Verification items for the finished model (mm, model axes). A direction names the side the tool comes from. Give positions to 0.01 mm unless a question says otherwise; leave off trailing zeros.
from build123d import *

# Parameters (mm, degrees)
SKETCH_2_R      = 2.5
EXTRUDE_1_DEPTH = 300


with BuildPart() as part:
    # 草图2 → 凸台-拉伸1 (new body)
    with BuildSketch(Plane.XY):
        with BuildLine():
            Line((-5.825824942, 5.993206118), (-5.825824942, 0.914526462))
            Line((-5.825824942, 0.914526462), (-8.786485114, -2.04613371))
            Line((-8.786485114, -2.04613371), (-10.425824942, -2.04613371))
            Line((-10.425824942, -2.04613371), (-10.425824942, 0.35386629))
            Line((-10.425824942, 0.35386629), (-11.425824942, 0.35386629))
            Line((-11.425824942, 0.35386629), (-11.425824942, -0.14613371))
            Line((-11.425824942, -0.14613371), (-12.225824942, -0.14613371))
            Line((-12.225824942, -0.14613371), (-12.225824942, -5.04613371))
            ThreePointArc((-12.225824942, -5.04613371), (-11.786485114, -6.106793882), (-10.725824942, -6.54613371))
            Line((-10.725824942, -6.54613371), (-5.825824942, -6.54613371))
            Line((-5.825824942, -6.54613371), (-5.825824942, -5.74613371))
            Line((-5.825824942, -5.74613371), (-5.325824942, -5.74613371))
            Line((-5.325824942, -5.74613371), (-5.325824942, -4.74613371))
            Line((-5.325824942, -4.74613371), (-7.725824942, -4.74613371))
            Line((-7.725824942, -4.74613371), (-7.725824942, -3.106793882))
            Line((-7.725824942, -3.106793882), (-4.765164771, -0.14613371))
            Line((-4.765164771, -0.14613371), (0.313514886, -0.14613371))
            Line((0.313514886, -0.14613371), (3.274175058, -3.106793882))
            Line((3.274175058, -3.106793882), (3.274175058, -4.74613371))
            Line((3.274175058, -4.74613371), (0.874175058, -4.74613371))
            Line((0.874175058, -4.74613371), (0.874175058, -5.74613371))
            Line((0.874175058, -5.74613371), (1.374175058, -5.74613371))
            Line((1.374175058, -5.74613371), (1.374175058, -6.54613371))
            Line((1.374175058, -6.54613371), (6.274175058, -6.54613371))
            ThreePointArc((6.274175058, -6.54613371), (7.334835229, -6.106793882), (7.774175058, -5.04613371))
            Line((7.774175058, -5.04613371), (7.774175058, -0.14613371))
            Line((7.774175058, -0.14613371), (6.974175058, -0.14613371))
            Line((6.974175058, -0.14613371), (6.974175058, 0.35386629))
            Line((6.974175058, 0.35386629), (5.974175058, 0.35386629))
            Line((5.974175058, 0.35386629), (5.974175058, -2.04613371))
            Line((5.974175058, -2.04613371), (4.334835229, -2.04613371))
            Line((4.334835229, -2.04613371), (1.374175058, 0.914526462))
            Line((1.374175058, 0.914526462), (1.374175058, 5.993206118))
            Line((1.374175058, 5.993206118), (4.334835229, 8.95386629))
            Line((4.334835229, 8.95386629), (5.974175058, 8.95386629))
            Line((5.974175058, 8.95386629), (5.974175058, 6.55386629))
            Line((5.974175058, 6.55386629), (6.974175058, 6.55386629))
            Line((6.974175058, 6.55386629), (6.974175058, 7.05386629))
            Line((6.974175058, 7.05386629), (7.774175058, 7.05386629))
            Line((7.774175058, 7.05386629), (7.774175058, 11.95386629))
            ThreePointArc((7.774175058, 11.95386629), (7.334835229, 13.014526462), (6.274175058, 13.45386629))
            Line((6.274175058, 13.45386629), (1.374175058, 13.45386629))
            Line((1.374175058, 13.45386629), (1.374175058, 12.65386629))
            Line((1.374175058, 12.65386629), (0.874175058, 12.65386629))
            Line((0.874175058, 12.65386629), (0.874175058, 11.65386629))
            Line((0.874175058, 11.65386629), (3.274175058, 11.65386629))
            Line((3.274175058, 11.65386629), (3.274175058, 10.014526462))
            Line((3.274175058, 10.014526462), (0.313514886, 7.05386629))
            Line((0.313514886, 7.05386629), (-4.765164771, 7.05386629))
            Line((-4.765164771, 7.05386629), (-7.725824942, 10.014526462))
            Line((-7.725824942, 10.014526462), (-7.725824942, 11.65386629))
            Line((-7.725824942, 11.65386629), (-5.325824942, 11.65386629))
            Line((-5.325824942, 11.65386629), (-5.325824942, 12.65386629))
            Line((-5.325824942, 12.65386629), (-5.825824942, 12.65386629))
            Line((-5.825824942, 12.65386629), (-5.825824942, 13.45386629))
            Line((-5.825824942, 13.45386629), (-10.725824942, 13.45386629))
            ThreePointArc((-10.725824942, 13.45386629), (-11.786485114, 13.014526462), (-12.225824942, 11.95386629))
            Line((-12.225824942, 11.95386629), (-12.225824942, 7.05386629))
            Line((-12.225824942, 7.05386629), (-11.425824942, 7.05386629))
            Line((-11.425824942, 7.05386629), (-11.425824942, 6.55386629))
            Line((-11.425824942, 6.55386629), (-10.425824942, 6.55386629))
            Line((-10.425824942, 6.55386629), (-10.425824942, 8.95386629))
            Line((-10.425824942, 8.95386629), (-8.786485114, 8.95386629))
            Line((-8.786485114, 8.95386629), (-5.825824942, 5.993206118))
        make_face()
        with Locations((-2.225824942, 3.45386629)):
            Circle(SKETCH_2_R, mode=Mode.SUBTRACT)
    extrude(amount=EXTRUDE_1_DEPTH)


solid = part.part
(1) Scan lines: line 1 (Y direction, x = 5.25, z = 118.5); line 2 (X direction, y = -4, z = 196.5); line 3 (Y direction, x = -2.75, z = 19.5). Record each from-to range of solid material in increasing order.
Solved:
line 1: y = -6.55 to -2.05, 8.95 to 13.45
line 2: x = -12.23 to -7.73, 3.27 to 7.77
line 3: y = -0.15 to 1.01, 5.9 to 7.05
(2) Set-up check for faces 1 (the flat face through (1.374, 3, 148)), 2 (the flat face through (-2, 7.054, 148)), 3 (the flat face through (7.774, -3, 148)), 4 (the flat face through (-5.826, 3, 148)): record each of +Z, -Z, +X, -X, +Y, -Y from which the full face is reachable in a straight line by a thin tool's end or side.
Solved:
face 1: +Z, -Z, +X
face 2: +Z, -Z, +Y
face 3: +Z, -Z, +X, +Y, -Y
face 4: +Z, -Z, -X
(3) Go/stop test with flat-tipped pins: pin 1 (0.5 mm diameter, centred on x = 6.5, z = 97, fed in from -Y); pin 2 (2.5 mm diameter, centred on y = 3, z = 102, fed in from -X); pin 3 (4 mm diameter, centred on x = -2.5, z = 168, fed in from -Y). Record where each tip stops, or that it passes through.
Solved:
pin 1: stops at y = -6.55
pin 2: stops at x = -5.83
pin 3: stops at y = -0.15
(4) Release check for a two-part mould opening along Y. For faces 5 (the cylindrical face through (-2.768, 1.013, 147.9)), 6 (the flat face through (-2, -0.146, 148)), 7 (the flat face through (-12.226, 10, 148)) record: pulls with the +Y half, pulls with the -Y half, needs draft (parallel to the pull), parting line crosses it, or undercut.
Solved:
face 5: undercut
face 6: pulls with the -Y half
face 7: needs draft
